Geometry: final body of the model. Coordinates: model frame, mm. Face numbers are marked on the shaded views. A direction names the side the tool comes from. Round coordinates to 2 decimals unless told otherwise and drop trailing zeros. Write each loop counter-clockwise with the first axis right and the second up, starting at its lowest first coordinate (ties: lowest second). Pieces come first, ordered by that corner, then holes.
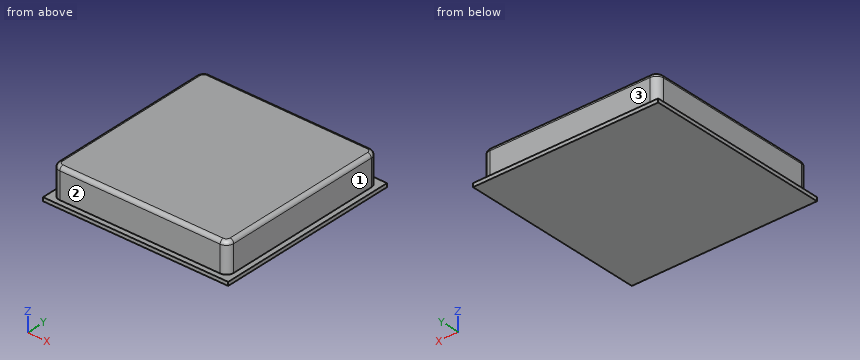
Autodesk Inventor part; units mm, degrees
ref_plane "YZ Plane" through (0, 0, 0) normal (1, 0, 0) x (0, 1, 0)
ref_plane "XZ Plane" through (0, 0, 0) normal (0, 1, 0) x (-1, 0, 0)
ref_plane "XY Plane" through (0, 0, 0) normal (0, 0, 1) x (1, 0, 0)
sketch "Sketch1" plane through (0, 0, 0) normal (0, 0, 1) x (1, 0, 0)
  line L0 (0, 0) -> (25.4, 0)
  line L1 (25.4, 0) -> (25.4, 25.4)
  line L2 (25.4, 25.4) -> (0, 25.4)
  line L3 (0, 25.4) -> (0, 0)
  dimension "d0" = 25.4
  dimension "d1" = 25.4
extrude "Extrusion1" add sketch "Sketch1" along normal blind 0.5
sketch "Sketch2" plane through (0, 0, 0) normal (0, 0, -1) x (-1, 0, 0)
  line L0 (-24.7, 0.7) -> (-0.7, 0.7)
  line L1 (-0.7, 0.7) -> (-0.7, 24.7)
  line L2 (-0.7, 24.7) -> (-24.7, 24.7)
  line L3 (-24.7, 24.7) -> (-24.7, 0.7)
  line L4 (-25.4, 25.4) -> (0, 25.4)
  line L5 (0, 25.4) -> (0, 0)
  point P0 (-12.7, 24.7)
  point P1 (-12.7, 25.4)
  point P2 (-0.7, 12.7)
  point P3 (0, 12.7)
  dimension "d4" = 24
  dimension "d5" = 24
extrude "Extrusion2" add sketch "Sketch2" against normal blind 4.6
fillet "Fillet1" radius 1 4 edges at (24.7, 24.7, 2.55) (0.7, 24.7, 2.55) (0.7, 0.7, 2.55) (24.7, 0.7, 2.55)
fillet "Fillet2" radius 0.5 8 edges at (24.4071, 24.4071, 4.6) (12.7, 24.7, 4.6) (0.9929, 24.4071, 4.6) (0.7, 12.7, 4.6) (0.9929, 0.9929, 4.6) (12.7, 0.7, 4.6) (24.4071, 0.9929, 4.6) (24.7, 12.7, 4.6)
properties part number "Rubber Square 1 in" material "ABS Plastic"
1) Section B-B on z = 2.8. Output: boundary loops of the cut face in (x, y).
2) Reachability of the marked faces 1, 2 and 3 from +Z, -Z, +X, -X, +Y, -Y: full face, straight path, thin tool, end or side. Return the list, or none.
3) First-contact query: P1, Ø1.8, axis at y = 14.5, z = 2, coming from the +X side; P2, Ø1, axis at y = 8, z = 3, coming from the -X side; P3, Ø1, axis at x = 7.5, z = 2.5, coming from the +Y side. Flat tips, straight axial feed; report the tip coordinate or a pass-through.
4) Section A-A on x = 5.5. Output: boundary loops of the cut face in (y, z), plus the area to 3 significant figures.
5) Line query: probe 1 along X at (y, z) = (2, 2.7); probe 2 along Y at (x, z) = (24.25, 0.9). Output: solid intervals per line, ascending.
Filled in:
1. outline: (0.7, 1.7) arc R1 ccw to (1.7, 0.7) - (23.7, 0.7) arc R1 ccw to (24.7, 1.7) - (24.7, 23.7) arc R1 ccw to (23.7, 24.7) - (1.7, 24.7) arc R1 ccw to (0.7, 23.7) - close
2. face 1: +Z, +X, +Y, -Y
2. face 2: +Z, +X, -X, -Y
2. face 3: +Z, +X, -X, +Y
3. P1: stops at x = 24.7
3. P2: stops at x = 0.7
3. P3: stops at y = 24.7
4. outline: (0, 0) - (25.4, 0) - (25.4, 0.5) - (24.7, 0.5) - (24.7, 4.1) arc R0.5 ccw to (24.2, 4.6) - (1.2, 4.6) arc R0.5 ccw to (0.7, 4.1) - (0.7, 0.5) - (0, 0.5) - close
4. area: 111 mm2
5. probe 1: x = 0.7 to 24.7
5. probe 2: y = 0.86 to 24.54
